```python
from build123d import *

# Parameters (mm, degrees)
SKETCH_1_W             = 136
SKETCH_1_H             = 104
EXTRUDE_1_DEPTH        = 10.5
SKETCH_1_3_W           = 106.4
SKETCH_1_3_H           = 68
SKETCH_1_3_W_2         = 81.4
SKETCH_1_3_H_2         = 15
CUT_EXTRUDE_1428_DEPTH = 4.3
CUT_EXTRUDE_1765_REACH = 173.529
SKETCH_4_W             = 15
SKETCH_4_H             = 35
CUT_EXTRUDE_3_DEPTH    = 3


with BuildPart() as part:
    # Sketch 1 → Extrude 1 (new body)
    with BuildSketch(Plane.XY):
        with Locations((68, 52)):
            Rectangle(SKETCH_1_W, SKETCH_1_H)
    extrude(amount=-EXTRUDE_1_DEPTH)

    # Sketch 1_3 → Cut-Extrude 1428 (cut)
    with BuildSketch(Plane.XY):
        with Locations((56.88, 49)):
            Rectangle(SKETCH_1_3_W, SKETCH_1_3_H)
        with Locations((54.38, 7.5)):
            Rectangle(SKETCH_1_3_W_2, SKETCH_1_3_H_2)
    extrude(amount=-CUT_EXTRUDE_1428_DEPTH, mode=Mode.SUBTRACT)

    # Sketch 1_5 → Cut-Extrude 1765 (cut, up to next)
    with BuildSketch(Plane.XY, mode=Mode.PRIVATE) as cut_extrude_1765_sk1:
        Polygon((7.133974596, 96.5), (8.866025404, 96.5), (9.732050808, 98), (8.866025404, 99.5), (7.133974596, 99.5), (6.267949192, 98), align=None)
    cut_extrude_1765_tool1 = extrude(cut_extrude_1765_sk1.sketch, amount=-CUT_EXTRUDE_1765_REACH, mode=Mode.PRIVATE) & part.part
    # Sketch 1_5 → Cut-Extrude 1765 (cut, up to next)
    with BuildSketch(Plane.XY, mode=Mode.PRIVATE) as cut_extrude_1765_sk2:
        Polygon((129.133974596, 96.5), (130.866025404, 96.5), (131.732050808, 98), (130.866025404, 99.5), (129.133974596, 99.5), (128.267949192, 98), align=None)
    cut_extrude_1765_tool2 = extrude(cut_extrude_1765_sk2.sketch, amount=-CUT_EXTRUDE_1765_REACH, mode=Mode.PRIVATE) & part.part
    # Sketch 1_5 → Cut-Extrude 1765 (cut, up to next)
    with BuildSketch(Plane.XY, mode=Mode.PRIVATE) as cut_extrude_1765_sk3:
        Polygon((130.866025404, 7.5), (129.133974596, 7.5), (128.267949192, 6), (129.133974596, 4.5), (130.866025404, 4.5), (131.732050808, 6), align=None)
    cut_extrude_1765_tool3 = extrude(cut_extrude_1765_sk3.sketch, amount=-CUT_EXTRUDE_1765_REACH, mode=Mode.PRIVATE) & part.part
    # Sketch 1_5 → Cut-Extrude 1765 (cut, up to next)
    with BuildSketch(Plane.XY, mode=Mode.PRIVATE) as cut_extrude_1765_sk4:
        Polygon((7.133974596, 4.5), (8.866025404, 4.5), (9.732050808, 6), (8.866025404, 7.5), (7.133974596, 7.5), (6.267949192, 6), align=None)
    cut_extrude_1765_tool4 = extrude(cut_extrude_1765_sk4.sketch, amount=-CUT_EXTRUDE_1765_REACH, mode=Mode.PRIVATE) & part.part
    # Sketch 1_5 → Cut-Extrude 1765 (cut, up to next)
    with BuildSketch(Plane.XY, mode=Mode.PRIVATE) as cut_extrude_1765_sk5:
        Polygon((101.133974596, 4.5), (102.866025404, 4.5), (103.732050808, 6), (102.866025404, 7.5), (101.133974596, 7.5), (100.267949192, 6), align=None)
    cut_extrude_1765_tool5 = extrude(cut_extrude_1765_sk5.sketch, amount=-CUT_EXTRUDE_1765_REACH, mode=Mode.PRIVATE) & part.part
    # Sketch 1_5 → Cut-Extrude 1765 (cut, up to next)
    with BuildSketch(Plane.XY, mode=Mode.PRIVATE) as cut_extrude_1765_sk6:
        Polygon((103.732050808, 98), (102.866025404, 99.5), (101.133974596, 99.5), (100.267949192, 98), (101.133974596, 96.5), (102.866025404, 96.5), align=None)
    cut_extrude_1765_tool6 = extrude(cut_extrude_1765_sk6.sketch, amount=-CUT_EXTRUDE_1765_REACH, mode=Mode.PRIVATE) & part.part
    add(cut_extrude_1765_tool1.solids().sort_by_distance((8, 98, 0))[0], mode=Mode.SUBTRACT)
    add(cut_extrude_1765_tool2.solids().sort_by_distance((130, 98, 0))[0], mode=Mode.SUBTRACT)
    add(cut_extrude_1765_tool3.solids().sort_by_distance((130, 6, 0))[0], mode=Mode.SUBTRACT)
    add(cut_extrude_1765_tool4.solids().sort_by_distance((8, 6, 0))[0], mode=Mode.SUBTRACT)
    add(cut_extrude_1765_tool5.solids().sort_by_distance((102, 6, 0))[0], mode=Mode.SUBTRACT)
    add(cut_extrude_1765_tool6.solids().sort_by_distance((102, 98, 0))[0], mode=Mode.SUBTRACT)

    # Sketch 4 → Cut-Extrude 3 (cut)
    with BuildSketch(Plane(origin=(0, 0, -10.5), x_dir=(-1, 0, 0), z_dir=(0, 0, -1))):
        with Locations((-12.767949192, 27)):
            Rectangle(SKETCH_4_W, SKETCH_4_H)
    extrude(amount=-CUT_EXTRUDE_3_DEPTH, mode=Mode.SUBTRACT)


solid = part.part
```
Here's how the part is built. I have some questions about the finished solid (model axes, mm). A direction names the side the tool comes from. Give positions to 0.01 mm unless a question says otherwise; leave off trailing zeros. Loops run counter-clockwise (first coordinate to the right, second up) from the corner with the lowest first, then second, coordinate; pieces in that order, holes last. Notation, with made-up numbers: M 8.5,-29 L 40.5,-29 A34 cw 40.5,4 Z; hole C 65.25,33.5 d8. An arc over 180 degrees is marked long. Use one line per item in the form item = value. Start each with the question number.
Q1. Which directions (+Z, -Z, +X, -X, +Y, -Y) give clear straight access to the entire face, cutting with the end or side of a thin tool? Please do faces 4 (the flat face through (136, 51, -5)), 5 (the flat face through (56, 83, -2)), 6 (the flat face through (5.268, 27, -9)), 7 (the flat face through (13.68, 7, -2)), 8 (the flat face through (67, 53, -10.5)).
Q2. Will these pins go through, and if not, where does the flat tip stop? pin 1 Ø1.5 at (x, y) = (30, 31) entering from +Z; pin 2 Ø4.5 at (x, y) = (15, 23.5) entering from -Z; pin 3 Ø3.5 at (x, z) = (46.5, -2.5) entering from -Y.
Q3. If we section it at A-A (y = 58.5): Write out the boundary of the cut face in (x, z), then the cut area to 3 significant figures.
Q4. If we section it at C-C (z = -2.75): State how many separate pieces and enclosed holes the cut face has, then the cut area to 3 significant figures.
Q5. Thinking about a two-plate mould opening in Y: for faces 1 (the flat face through (67, 104, -5)), 2 (the flat face through (102, 15, -2)), 3 (the flat face through (97, 87, 0)), which applies, +Y half, -Y half, draft (parallel to the pull), parting line (faces both ways), or undercut?
Q6. If we section it at B-B (x = 107): Write out the boundary of the cut face in (y, z).
Q7. I need wall thicknesses on line 1 along X through (y, z) = (6, -1); line 2 along X through (y, z) = (19, -1.5); line 3 along Y through (x, z) = (10.5, -8). Which ranges of each line are inside material? Lowest first, please.
Q8. If we section it at D-D (y = 12.5): Write out the boundary of the cut face in (x, z), then the cut area to 3 significant figures.
Taken from the geometry:
q1.face_4 = +Z, -Z, +X, +Y, -Y
q1.face_5 = +Z
q1.face_6 = -Z
q1.face_7 = +Z, -Y
q1.face_8 = -Z, +X, -X, +Y, -Y
q2.pin_1 = -4.3
q2.pin_2 = -7.5
q2.pin_3 = 83
q3.outline = M 0,-10.5 L 136,-10.5 L 136,0 L 110.08,0 L 110.08,-4.3 L 3.68,-4.3 L 3.68,0 L 0,0 Z
q3.area = 970 mm^2
q4.separate_pieces = 1
q4.enclosed_holes = 6
q4.area = 5,640 mm^2
q5.face_1 = +Y half
q5.face_2 = undercut
q5.face_3 = draft
q6.outline = M 0,-10.5 L 104,-10.5 L 104,0 L 83,0 L 83,-4.3 L 15,-4.3 L 15,0 L 0,0 Z
q7.line_1 = 0 to 6.27, 9.73 to 13.68, 95.08 to 100.27, 103.73 to 128.27, 131.73 to 136
q7.line_2 = 0 to 3.68, 110.08 to 136
q7.line_3 = 0 to 9.5, 44.5 to 104
q8.outline = M 0,-10.5 L 5.27,-10.5 L 5.27,-7.5 L 20.27,-7.5 L 20.27,-10.5 L 136,-10.5 L 136,0 L 95.08,0 L 95.08,-4.3 L 13.68,-4.3 L 13.68,0 L 0,0 Z
q8.area = 1,030 mm^2
